Autodesk Inventor part; units mm, degrees
ref_plane "YZ Plane" through (0, 0, 0) normal (1, 0, 0) x (0, 1, 0)
ref_plane "XZ Plane" through (0, 0, 0) normal (0, 1, 0) x (-1, 0, 0)
ref_plane "XY Plane" through (0, 0, 0) normal (0, 0, 1) x (1, 0, 0)
sketch "Sketch1" plane through (0, 0, 0) normal (0, 0, 1) x (1, 0, 0)
  line L0 (-70, -20) -> (70, -20)
  line L1 (70, -20) -> (70, 20)
  line L2 (70, 20) -> (-70, 20)
  line L3 (-70, 20) -> (-70, -20)
  line L4 (-70, -20) -> (70, 20) construction
  line L5 (70, -20) -> (-70, 20) construction
  point P0 (0, 0)
  dimension "d0" = 140
  dimension "d1" = 40
extrude "Extrusion1" add sketch "Sketch1" along normal blind 6.35
sketch "Sketch2" plane through (0, 0, 0) normal (0, 0, -1) x (-1, 0, 0)
  circle A0 centre (-50, 0) radius 4
  circle A1 centre (0, 10) radius 4
  circle A2 centre (50, 0) radius 4
  line L0 (-70, -20) -> (-70, 20)
  point P0 (0, 0)
  point P1 (-70, 0)
  dimension "d4" = 20
  dimension "d5" = 100
  dimension "d6" = 50
  dimension "d7" = 8
  dimension "d8" = 10
extrude "Extrusion2" cut sketch "Sketch2" against normal through all
thicken "Thicken1" operation add thickness 5 both sides no extend neighbours yes toward (0, 1, 0) faces at (23.3333, 20, 2.1167)
properties part number "Zapata_freno"
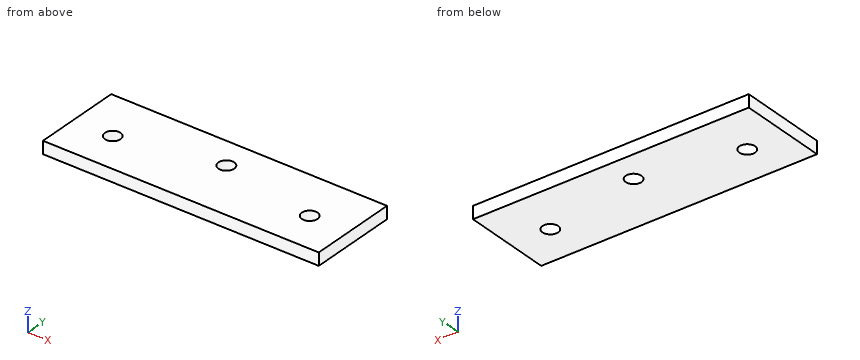
Design review of the part built by this model. Coordinates are the model's own, in mm. Coordinates: 2 decimals unless noted, no trailing zeros. Loops run counter-clockwise (first coordinate to the right, second up) from the corner with the lowest first, then second, coordinate; pieces in that order, holes last. Notation, with made-up numbers: (-13, 49) - (0, 49) arc R21 ccw to (0, 79) - close; hole circle Ø3 at (-11.5, -4). An arc over 180 degrees is marked (long way). Use CSV: the item, a comma, the result in double quotes. Start each with the question number.
1. Add section D-D on z = 1. Give the boundary of the cut face in (x, y).
2. To check wall thickness, follow probe 1 along Y at (x, z) = (0, 2); probe 2 along Y at (x, z) = (-50, 3.75); probe 3 along X at (y, z) = (12.5, 4.5). State the ranges of each line that lie inside material, in increasing order.
3. Add section B-B on y = 0. Give the boundary of the cut face in (x, z).
4. Add section C-C on x = 1.5. Give the boundary of the cut face in (y, z).
5. Add section A-A on y = 10. Give the boundary of the cut face in (x, z).
Resolved:
1,outline,"(-70, -20) - (70, -20) - (70, 25) - (-70, 25) - close; hole circle Ø8 at (-50, 0); hole circle Ø8 at (0, 10); hole circle Ø8 at (50, 0)"
2,probe 1,"-20 to 6, 14 to 25"
2,probe 2,"-20 to -4, 4 to 25"
2,probe 3,"-70 to -3.12, 3.12 to 70"
3,outline,"(-70, 0) - (-54, 0) - (-54, 6.35) - (-70, 6.35) - close; (-46, 0) - (46, 0) - (46, 6.35) - (-46, 6.35) - close; (54, 0) - (70, 0) - (70, 6.35) - (54, 6.35) - close"
4,outline,"(-20, 0) - (6.29, 0) - (6.29, 6.35) - (-20, 6.35) - close; (13.71, 0) - (25, 0) - (25, 6.35) - (13.71, 6.35) - close"
5,outline,"(-70, 0) - (-4, 0) - (-4, 6.35) - (-70, 6.35) - close; (4, 0) - (70, 0) - (70, 6.35) - (4, 6.35) - close"
